```python
from build123d import *

# Parameters (mm, degrees)
ESBO_O1_R                = 80
RESSALTO_EXTRUS_O1_DEPTH = 130
ESBO_O2_R                = 60
CORTE_EXTRUS_O1_DEPTH    = 100
ESBO_O4_W                = 5
ESBO_O4_H                = 5
VARREDURA2_PROFILE_R     = 10
VARREDURA3_PROFILE_R     = 10


with BuildPart() as part:
    # Esboço1 → Ressalto-extrusão1 (new body)
    with BuildSketch(Plane(origin=(0, 0, 0), x_dir=(1, 0, 0), z_dir=(0, 1, 0))):
        with Locations(Location((0, 0, 0), (0, 0, 270))):
            Circle(ESBO_O1_R)
    extrude(amount=RESSALTO_EXTRUS_O1_DEPTH)

    # Esboço2 → Corte-extrusão1 (cut)
    with BuildSketch(Plane(origin=(0, 130, 0), x_dir=(1, 0, 0), z_dir=(0, 1, 0))):
        with Locations(Location((0, 0, 0), (0, 0, 270))):
            Circle(ESBO_O2_R)
    extrude(amount=-CORTE_EXTRUS_O1_DEPTH, mode=Mode.SUBTRACT)

    # Esboço4 → Revolução1 (revolve)
    with BuildSketch(Plane(origin=(0, 0, 0), x_dir=(0, 0, -1), z_dir=(1, 0, 0))):
        with Locations((-70, 132.5)):
            Rectangle(ESBO_O4_W, ESBO_O4_H)
    revolve(axis=Axis((0, 130, 0), (0, -1, 0)))

    # Varredura2: sweep along a path in Esboço6
    with BuildLine(Plane.XY) as varredura2_path:
        Line((70, 107), (102, 107))
        ThreePointArc((102, 107), (112.606601718, 102.606601718), (117, 92))
        Line((117, 92), (117, 38))
        ThreePointArc((117, 38), (112.606601718, 27.393398282), (102, 23))
        Line((102, 23), (70, 23))
    # Varredura2 profile (on start of the path) → Varredura2 (sweep)
    with BuildSketch(Plane(origin=(70, 107, 0), x_dir=(0, 0, 1), z_dir=(1, 0, 0))):
        Circle(VARREDURA2_PROFILE_R)
    sweep(path=varredura2_path.line)

    # Varredura3: sweep along a path in Esboço36
    with BuildLine(Plane.XY) as varredura3_path:
        Line((-70, 107), (-102, 107))
        ThreePointArc((-102, 107), (-112.606601718, 102.606601718), (-117, 92))
        Line((-117, 92), (-117, 38))
        ThreePointArc((-117, 38), (-112.606601718, 27.393398282), (-102, 23))
        Line((-102, 23), (-70, 23))
    # Varredura3 profile (on start of the path) → Varredura3 (sweep)
    with BuildSketch(Plane(origin=(-70, 107, 0), x_dir=(0, 0, -1), z_dir=(-1, 0, 0))):
        Circle(VARREDURA3_PROFILE_R)
    sweep(path=varredura3_path.line)


solid = part.part
```
For this review, take the finished solid that the model builds, in its own axes (mm). A direction names the side the tool comes from. Round coordinates to 2 decimals unless told otherwise and drop trailing zeros. Order: outer loops, then holes, each group sorted by start corner. A loop starts at its lowest first (then second) coordinate and runs counter-clockwise, first axis right, second up. Notation, with made-up numbers: (-29, -39.5) -> (16, -39.5) arc R27 cw to (16, -4.5) -> close; hole circle Ø9 at (51.5, -1.5). An arc over 180 degrees is marked (long way). Use a Markdown table: item, result.
Item 1: For pin 1 (10 mm diameter, centred on x = 56, y = 17.5, fed in from -Z); pin 2 (12 mm diameter, centred on x = 55, y = 79, fed in from +Z); pin 3 (10 mm diameter, centred on x = 15.5, y = 48, fed in from +Z), all flat-tipped, find the tip position at first contact; note any pin that passes through.
Resolved:
| item | result |
|---|---|
| pin 1 | stops at z = -61.64 |
| pin 2 | stops at z = 63.24 |
| pin 3 | stops at z = 79.31 |
Item 2: Take a section at D-D (z = 0). State how many separate pieces and enclosed holes the cut face has, plus the area to 3 significant figures.
Resolved:
| item | result |
|---|---|
| separate pieces | 1 |
| enclosed holes | 2 |
| area | 14,700 mm² |
Item 3: Machinability: for faces 4 (the flat face through (1, 0, -1)), 5 (the flat face through (1, 30, -1)), 6 (the cylindrical face through (90.845, 97.085, -1.302)), which of the approach directions +Z, -Z, +X, -X, +Y, -Y give a long, thin tool a straight path to every point of the face, cutting with its end or side? Answer none if there is none.
Resolved:
| item | result |
|---|---|
| face 4 | +Z, -Z, +X, -X, -Y |
| face 5 | +Y |
| face 6 | none |
Item 4: For line 1 along Z through (x, y) = (0, 131.3); line 2 along X through (y, z) = (76.5, 0); line 3 along X through (y, z) = (96, 0), list the stretches that pass through material, from the lowest coordinate up. Write a range as [from, to].
Resolved:
| item | result |
|---|---|
| line 1 | z = [-72.5, -67.5], [67.5, 72.5] |
| line 2 | x = [-127, -107], [-80, -60], [60, 80], [107, 127] |
| line 3 | x = [-126.68, -105], [-80, -60], [60, 80], [105, 126.68] |
Item 5: Draft analysis for pull direction Y (two halves, no side actions). For faces 1 (the cylindrical face through (-90.528, 32.915, 1.302)), 2 (the flat face through (60, 130, -42)), 3 (the cylindrical face through (41.07, 132.54, -53.57)), state which applies: +Y half, -Y half, draft (parallel to the pull), parting line (faces both ways), or undercut.
Resolved:
| item | result |
|---|---|
| face 1 | undercut |
| face 2 | +Y half |
| face 3 | draft |
Item 6: Take a section at B-B (x = -83). State the section outline as (y, z) points.
Resolved:
| item | result |
|---|---|
| outline | circle Ø20 at (23, 0); circle Ø20 at (107, 0) |
Item 7: Take a section at C-C (y = 123.5). State the section outline as (x, z) points, plus the area to 3 significant figures.
Resolved:
| item | result |
|---|---|
| outline | circle Ø160 at (0, 0); hole circle Ø120 at (0, 0) |
| area | 8,800 mm² |
Item 8: Take a section at A-A (y = 83.5). State the section outline as (x, z) points, plus the area to 3 significant figures.
Resolved:
| item | result |
|---|---|
| outline | circle Ø20 at (-117, 0); circle Ø160 at (0, 0); circle Ø20 at (117, 0); hole circle Ø120 at (0, 0) |
| area | 9,420 mm² |
